The listing builds one solid part. Answer for the finished solid, in the listing's coordinates (mm). Face numbers are marked on the shaded views. A direction names the side the tool comes from. Round coordinates to 2 decimals unless told otherwise and drop trailing zeros. Loops run counter-clockwise (first coordinate to the right, second up) from the corner with the lowest first, then second, coordinate; pieces in that order, holes last. Notation, with made-up numbers: (-34.75, 29.5) - (20.25, 29.5) arc R21 ccw to (20.25, 56.5) - close; hole circle Ø9 at (7, 36). An arc over 180 degrees is marked (long way). One line per item, written item: value.
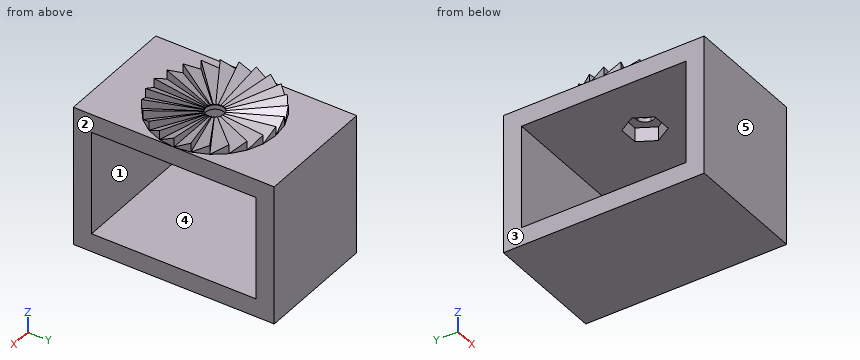
```python
from build123d import *

# Parameters (mm, degrees)
F5_COUNT      = 24
F6_W          = 33
F6_H          = 23
F6_W_2        = 27
F6_H_2        = 17
F7_DEPTH      = 10
F7_DEPTH_BACK = 10
F8_DEPTH      = 3
F8_DEPTH_BACK = 5
F10_DEPTH     = 2.3


with BuildPart() as f3:
    # F2 (on line) → F3 section 0
    with BuildSketch(Plane(origin=(1.2938400436, 9.8296975, 0), x_dir=(-0.9914483093, 0.1305, 0), z_dir=(0.1305, 0.9914483093, 0)), mode=Mode.PRIVATE) as f3_s0:
        Polygon((-1.3041549828, 0), (1.3058450172, 0), (1.3058450172, 1.5), align=None)
    loft([f3_s0.sketch, Vertex(0, 0, 0)])

    # F5: F3 ×24 about axis
    f5_axis = Axis((0, 0, 1.9288011827), (0, 0, 1))


with BuildPart() as f3_1:
    add(f3.part)
    for i in range(1, F5_COUNT):
        add(f3.part.rotate(f5_axis, i * 360 / F5_COUNT))

    # F6 (on Right) → F7 (join, two sides)
    with BuildSketch(Plane.YZ) as f7_sk:
        with Locations((0, -11.5)):
            Rectangle(F6_W, F6_H)
        with Locations((0, -11.5)):
            Rectangle(F6_W_2, F6_H_2, mode=Mode.SUBTRACT)
    extrude(amount=F7_DEPTH)
    extrude(f7_sk.sketch, amount=-F7_DEPTH_BACK)

    # F0 (on Top) → F8 (cut, two sides)
    with BuildSketch(Plane.XY) as f8_sk:
        with BuildLine():
            ThreePointArc((1.5, 0), (1.1900058865, 0.9131735816), (0.3881520131, 1.44890925))
            Line((0.3881520131, 1.44890925), (0, 0))
            Line((0, 0), (0, 1.5))
            ThreePointArc((0, 1.5), (-1.0606601718, -1.0606601718), (1.5, 0))
        make_face()
        with BuildLine():
            Line((0, 0), (0.3881520131, 1.44890925))
            ThreePointArc((0.3881520131, 1.44890925), (0.19575, 1.4871724639), (0, 1.5))
            Line((0, 1.5), (0, 0))
        make_face()
    extrude(amount=-F8_DEPTH, mode=Mode.SUBTRACT)
    extrude(f8_sk.sketch, amount=F8_DEPTH_BACK, mode=Mode.SUBTRACT)

    # F9 (on face) → F10 (cut)
    with BuildSketch(Plane(origin=(0, 0, -3), x_dir=(1, 0, 0), z_dir=(0, 0, -1))):
        Polygon((-3.1751729007, -0.0401295912), (-1.5528332049, -2.769845189), (1.6223396958, -2.7297155978), (3.1751729007, 0.0401295912), (1.5528332049, 2.769845189), (-1.6223396958, 2.7297155978), align=None)
    extrude(amount=-F10_DEPTH, mode=Mode.SUBTRACT)


solid = f3_1.part
```
1) For a pull along Y with two mould halves and no side action, classify the marked faces 3, 4 and 5 as released by +Y, released by -Y, zero draft, split by the parting line, or undercut.
Final values:
face 3: zero draft
face 4: undercut
face 5: released by -Y
2) A cutting plane is placed at B-B on y = 12. Give the vertices of the cut face in (x, z).
Final values:
outline: (-10, -23) - (10, -23) - (10, -20) - (-10, -20) - close; (-10, -3) - (10, -3) - (10, 0) - (-10, 0) - close
3) A cutting plane is placed at A-A on z = -9. Give the vertices of the cut face in (x, y).
Final values:
outline: (-10, -16.5) - (10, -16.5) - (10, -13.5) - (-10, -13.5) - close; (-10, 13.5) - (10, 13.5) - (10, 16.5) - (-10, 16.5) - close
4) For the marked faces 1 and 2, determine the directions among +Z, -Z, +X, -X, +Y, -Y from which every point of the face is accessible in a straight line to the end or side of a thin tool.
Final values:
face 1: +X, -X
face 2: +Z, -Z, +X, +Y, -Y
5) Consider L1, parallel to Y at x = 0, z = -0.3; L2, parallel to Y at x = 0.25, z = -5.75; L3, parallel to Z at x = 6.25, y = 10.5. Determine where each line is inside the solid, lowest interval first.
Final values:
L1: -16.5 to -1.5, 1.5 to 16.5
L2: -16.5 to -13.5, 13.5 to 16.5
L3: -23 to -20, -3 to 0
6) Each of these flat-tipped pins is pushed along its axis until it touches: pin 1 Ø10 at (x, y) = (-0.5, 2.5) entering from +Z; pin 2 Ø1.2 at (x, z) = (7, 1) entering from +Y; pin 3 Ø1 at (y, z) = (-11.5, -11) entering from +X; pin 4 Ø0.8 at (y, z) = (-7, 1) entering from +X. Where does it stop, or does it pass through?
Final values:
pin 1: z = 1.13
pin 2: y = 7.07
pin 3: through
pin 4: x = 7.07
